Geometry check sheet. Reference: the model listing, model coordinates, mm. A direction names the side the tool comes from. Round coordinates to 2 decimals unless told otherwise and drop trailing zeros. Order: outer loops, then holes, each group sorted by start corner. A loop starts at its lowest first (then second) coordinate and runs counter-clockwise, first axis right, second up.
(1) Cross-section at C-C on z = 28. Enter the section's corners in (x, y), and give its area (3 significant figures).
(2) Thickness scan on L1, parallel to Z at x = 95, y = 9; L2, parallel to X at y = -19, z = 24.5. Record the ranges inside material, lowest first.
(3) Cross-section at A-A on x = 71.5. Enter the section's corners in (y, z).
(4) Gauge pin test, flat ends, axial feed: P1, Ø1, axis at y = 10.5, z = 6, coming from the -X side; P2, Ø4, axis at x = 147, y = 15.5, coming from the +Z side; P3, Ø1, axis at y = -13, z = 16.5, coming from the -X side. Record the tip position at first contact, or that the pin passes through.
(5) Draft check along Z on faces 4 (the face through (148, 35, 0)), 5 (the face through (10, 0, 0)), 6 (the face through (148, 0, 35)). Enter one of: pulls with the +Z half, pulls with the -Z half, needs draft (parallel to the pull), parting line crosses it, or undercut.
(6) Set-up check for faces 1 (the face through (2.85, -0.07, -31.99)), 2 (the face through (44.643, -3.252, 29.93)), 3 (the face through (284.297, 18.986, -0.35)): record each of +Z, -Z, +X, -X, +Y, -Y from which the full face is reachable in a straight line by a thin tool's end or side.
(7) Cross-section at B-B on y = 0. Enter the section's corners in (x, z).
from build123d import *

# Parameters (mm, degrees)
SKETCH2_W           = 70
SKETCH2_H           = 70
BOSS_EXTRUDE1_DEPTH = 300
FILLET1_R           = 30
FILLET2_R           = 10
SHELL1_START        = -25
SHELL1_DEPTH        = 50
SKETCH3_R           = 15
BOSS_EXTRUDE2_DEPTH = 15
CUT_EXTRUDE1_START  = -30
SKETCH4_R           = 15
CUT_EXTRUDE1_DEPTH  = 30


# Read off the part's stored shape, not the designer's step: Shell1
with BuildPart() as part:
    # Sketch2 → Boss-Extrude1 (new body)
    with BuildSketch(Plane(origin=(0, 0, 0), x_dir=(0, 0, -1), z_dir=(1, 0, 0))):
        Rectangle(SKETCH2_W, SKETCH2_H)
    extrude(amount=BOSS_EXTRUDE1_DEPTH)

    # Fillet1
    fillet1_edges = [part.edges().sort_by_distance(p)[0] for p in [
        (300, 35, 0),
        (0, 35, 0),
        (0, -35, 0),
        (300, -35, 0),
    ]]
    fillet(fillet1_edges, radius=FILLET1_R)

    # Fillet2
    fillet2_edges = [part.edges().sort_by_distance(p)[0] for p in [
        (150, -35, -35),
        (150, -35, 35),
        (0, 0, -35),
        (150, 35, -35),
        (300, 0, -35),
        (291.213203436, 26.213203436, -35),
        (291.213203436, -26.213203436, -35),
        (8.786796564, 26.213203436, -35),
        (8.786796564, -26.213203436, -35),
        (0, 0, 35),
        (300, 0, 35),
        (150, 35, 35),
        (291.213203436, 26.213203436, 35),
        (291.213203436, -26.213203436, 35),
        (8.786796564, 26.213203436, 35),
        (8.786796564, -26.213203436, 35),
    ]]
    fillet(fillet2_edges, radius=FILLET2_R)

    # Shell1 outline → Shell1 (cut)
    with BuildSketch(Plane.XY.offset(SHELL1_START)):
        with BuildLine():
            Line((30, -25), (270, -25))
            ThreePointArc((270, -25), (284.142135624, -19.142135624), (290, -5))
            Line((290, -5), (290, 5))
            ThreePointArc((290, 5), (284.142135624, 19.142135624), (270, 25))
            Line((270, 25), (30, 25))
            ThreePointArc((30, 25), (15.857864376, 19.142135624), (10, 5))
            Line((10, 5), (10, -5))
            ThreePointArc((10, -5), (15.857864376, -19.142135624), (30, -25))
        make_face()
    extrude(amount=SHELL1_DEPTH, mode=Mode.SUBTRACT)

    # Sketch3 → Boss-Extrude2 (add)
    with BuildSketch(Plane.XY.offset(35)):
        with Locations(Location((30, 0, 0), (0, 0, 90))):
            Circle(SKETCH3_R)
        with Locations(Location((270, 0, 0), (0, 0, 90))):
            Circle(SKETCH3_R)
    extrude(amount=BOSS_EXTRUDE2_DEPTH)

    # Sketch4 → Cut-Extrude1 (cut)
    with BuildSketch(Plane.XY.offset(50).offset(CUT_EXTRUDE1_START)):
        with Locations(Location((30, 0, 0), (0, 0, 90))):
            Circle(SKETCH4_R)
    extrude(amount=CUT_EXTRUDE1_DEPTH, mode=Mode.SUBTRACT)


solid = part.part
Found:
1. outline: (0.46, -5) arc R29.54 ccw to (30, -34.54) - (270, -34.54) arc R29.54 ccw to (299.54, -5) - (299.54, 5) arc R29.54 ccw to (270, 34.54) - (30, 34.54) arc R29.54 ccw to (0.46, 5) - close; hole circle Ø30 at (30, 0)
1. area: 19,200 mm2
2. L1: z = -35 to -25, 25 to 35
2. L2: x = 3.47 to 15.72, 284.28 to 296.53
3. outline: (-35, -25) arc R10 ccw to (-25, -35) - (25, -35) arc R10 ccw to (35, -25) - (35, 25) arc R10 ccw to (25, 35) - (-25, 35) arc R10 ccw to (-35, 25) - close; hole (-25, -25) - (25, -25) - (25, 25) - (-25, 25) - close
4. P1: stops at x = 0.42
4. P2: stops at z = 35
4. P3: stops at x = 0.95
5. face 4: needs draft
5. face 5: undercut
5. face 6: pulls with the +Z half
6. face 1: -Z, -X, +Y, -Y
6. face 2: +Z
6. face 3: none
7. outline: (0, -25) arc R10 ccw to (10, -35) - (290, -35) arc R10 ccw to (300, -25) - (300, 25) arc R10 ccw to (290, 35) - (285, 35) - (285, 50) - (255, 50) - (255, 35) - (45, 35) - (45, 25) - (290, 25) - (290, -25) - (10, -25) - (10, 25) - (15, 25) - (15, 35) - (10, 35) arc R10 ccw to (0, 25) - close
